from build123d import *

# Parameters (mm, degrees)
SKETCH2_W            = 53
SKETCH2_H            = 9
BOSS_EXTRUDE1_DEPTH  = 3
SKETCH11_W           = 2
SKETCH11_H           = 9
CUT_EXTRUDE3_DEPTH   = 5
SKETCH12_W           = 3
SKETCH12_H           = 9
BOSS_EXTRUDE7_DEPTH  = 1
SKETCH13_W           = 1
SKETCH13_H           = 1
BOSS_EXTRUDE8_DEPTH  = 4
SKETCH14_W           = 1
SKETCH14_H           = 1
BOSS_EXTRUDE9_DEPTH  = 5
SKETCH15_W           = 45.862173985
SKETCH15_H           = 3
BOSS_EXTRUDE10_DEPTH = 1.5
SKETCH25_W           = 3
SKETCH25_H           = 9
BOSS_EXTRUDE13_DEPTH = 1
SKETCH24_R           = 1.16794594
CUT_EXTRUDE7_DEPTH   = 9
SKETCH26_W           = 0.9784551
SKETCH26_H           = 1.939455742
CUT_EXTRUDE8_DEPTH   = 9
SKETCH27_W           = 45.862173985
SKETCH27_H           = 3
BOSS_EXTRUDE14_DEPTH = 2
SKETCH28_W           = 41.224865511
SKETCH28_H           = 1
CUT_EXTRUDE9_DEPTH   = 1.5
SKETCH29_W           = 3
SKETCH29_H           = 12.5
BOSS_EXTRUDE15_DEPTH = 1
BOSS_EXTRUDE16_DEPTH = 1
SKETCH31_W           = 2.328454802
SKETCH31_H           = 1
CUT_EXTRUDE10_DEPTH  = 1.5
BOSS_EXTRUDE17_DEPTH = 2
BOSS_EXTRUDE18_REACH = 53.942
SKETCH34_W           = 46.86
SKETCH34_H           = 1.5
SKETCH35_W           = 43.553320313
SKETCH35_H           = 1.25
CUT_EXTRUDE11_DEPTH  = 1
CUT_EXTRUDE12_REACH  = 54.259
SKETCH36_W           = 46.86
SKETCH36_H           = 3.75
SKETCH37_W           = 2
SKETCH37_H           = 2.25
CUT_EXTRUDE13_DEPTH  = 10
BOSS_EXTRUDE19_DEPTH = 2.5
SKETCH42_W           = 43.553320313
SKETCH42_H           = 1
BOSS_EXTRUDE20_DEPTH = 1
SKETCH44_W           = 46.862173985
SKETCH44_H           = 1
BOSS_EXTRUDE21_DEPTH = 5
SKETCH46_W           = 43.553320313
SKETCH46_H           = 1
BOSS_EXTRUDE22_DEPTH = 1


with BuildPart() as part:
    # Sketch2 → Boss-Extrude1 (new body)
    with BuildSketch(Plane.XY):
        with Locations((26.5, 4.5)):
            Rectangle(SKETCH2_W, SKETCH2_H)
    extrude(amount=BOSS_EXTRUDE1_DEPTH)

    # Sketch11 → Cut-Extrude3 (cut)
    with BuildSketch(Plane.XY.offset(3)):
        with Locations((52, 4.5)):
            Rectangle(SKETCH11_W, SKETCH11_H)
    extrude(amount=-CUT_EXTRUDE3_DEPTH, mode=Mode.SUBTRACT)

    # Sketch12 → Boss-Extrude7 (add)
    with BuildSketch(Plane.XY.offset(3)):
        with Locations((48, 4.5)):
            Rectangle(SKETCH12_W, SKETCH12_H)
    extrude(amount=BOSS_EXTRUDE7_DEPTH)

    # Sketch13 → Boss-Extrude8 (add)
    with BuildSketch(Plane.XY.offset(3)):
        with Locations((7, 7.5)):
            Rectangle(SKETCH13_W, SKETCH13_H)
        with Locations((7, 1.5)):
            Rectangle(SKETCH13_W, SKETCH13_H)
    extrude(amount=BOSS_EXTRUDE8_DEPTH)

    # Sketch14 → Boss-Extrude9 (add)
    with BuildSketch(Plane.XZ.offset(-7)):
        with Locations((7, 6.5)):
            Rectangle(SKETCH14_W, SKETCH14_H)
    extrude(amount=BOSS_EXTRUDE9_DEPTH)

    # Sketch15 → Boss-Extrude10 (add)
    with BuildSketch(Plane.XZ):
        with Locations((22.931086993, 1.5)):
            Rectangle(SKETCH15_W, SKETCH15_H)
    extrude(amount=BOSS_EXTRUDE10_DEPTH)

    # Sketch25 → Boss-Extrude13 (add)
    with BuildSketch(Plane(origin=(0, 0, 0), x_dir=(-1, 0, 0), z_dir=(0, 0, -1))):
        with Locations((-48, 4.5)):
            Rectangle(SKETCH25_W, SKETCH25_H)
    extrude(amount=BOSS_EXTRUDE13_DEPTH)

    # Sketch24 → Cut-Extrude7 (cut)
    with BuildSketch(Plane(origin=(0, 9, 0), x_dir=(1, 0, 0), z_dir=(0, 1, 0))):
        with Locations(Location((48, -2, 0), (0, 0, 270))):
            Circle(SKETCH24_R)
    extrude(amount=-CUT_EXTRUDE7_DEPTH, mode=Mode.SUBTRACT)

    # Sketch26 → Cut-Extrude8 (cut)
    with BuildSketch(Plane(origin=(0, 9, 0), x_dir=(1, 0, 0), z_dir=(0, 1, 0))):
        with Locations((48, 0.030272129)):
            Rectangle(SKETCH26_W, SKETCH26_H)
    extrude(amount=-CUT_EXTRUDE8_DEPTH, mode=Mode.SUBTRACT)

    # Sketch27 → Boss-Extrude14 (add)
    with BuildSketch(Plane.XZ.offset(1.5)):
        with Locations((22.931086993, 1.5)):
            Rectangle(SKETCH27_W, SKETCH27_H)
    extrude(amount=BOSS_EXTRUDE14_DEPTH)

    # Sketch28 → Cut-Extrude9 (cut)
    with BuildSketch(Plane.XZ.offset(3.5)):
        with Locations((22.921286428, 0.5)):
            Rectangle(SKETCH28_W, SKETCH28_H)
    extrude(amount=-CUT_EXTRUDE9_DEPTH, mode=Mode.SUBTRACT)

    # Sketch29 → Boss-Extrude15 (add)
    with BuildSketch(Plane.ZY):
        with Locations((1.5, 2.75)):
            Rectangle(SKETCH29_W, SKETCH29_H)
    extrude(amount=BOSS_EXTRUDE15_DEPTH)

    # Sketch30 → Boss-Extrude16 (add)
    with BuildSketch(Plane.ZY.offset(-6.5)):
        Polygon((3, 8), (3, 7), (6, 7), (6, 2), (3, 2), (3, 1), (7, 1), (7, 8), align=None)
    extrude(amount=BOSS_EXTRUDE16_DEPTH)

    # Sketch31 → Cut-Extrude10 (cut)
    with BuildSketch(Plane.XZ.offset(3.5)):
        with Locations((44.697946584, 0.5)):
            Rectangle(SKETCH31_W, SKETCH31_H)
    extrude(amount=-CUT_EXTRUDE10_DEPTH, mode=Mode.SUBTRACT)

    # Sketch32 → Boss-Extrude17 (add)
    with BuildSketch(Plane.XZ.offset(3.5)):
        Polygon((-1, 3), (-1, 0), (2.308853672, 0), (2.308853672, 1), (45.862173985, 1), (45.862173985, 3), align=None)
    extrude(amount=BOSS_EXTRUDE17_DEPTH)

    # Boss-Extrude18: up to this face of the body (flat: up to its plane)
    boss_extrude18_end = Plane(part.part.faces().sort_by_distance((22.213634354, 3.353188918, 0))[0])
    # Sketch34 → Boss-Extrude18 (add, up to the picked face)
    with BuildSketch(Plane.XY.offset(3), mode=Mode.PRIVATE) as boss_extrude18_sk1:
        with Locations((22.43, -6.25)):
            Rectangle(SKETCH34_W, SKETCH34_H)
    boss_extrude18_tool1 = split(extrude(boss_extrude18_sk1.sketch, amount=-BOSS_EXTRUDE18_REACH, mode=Mode.PRIVATE), bisect_by=boss_extrude18_end, keep=Keep.BOTH, mode=Mode.PRIVATE)
    add(boss_extrude18_tool1.solids().sort_by(Axis((22.43, -6.25, 3), (0, 0, -1)))[0])

    # Sketch35 → Cut-Extrude11 (cut)
    with BuildSketch(Plane(origin=(0, 0, 0), x_dir=(-1, 0, 0), z_dir=(0, 0, -1))):
        with Locations((-24.085513829, -1.375)):
            Rectangle(SKETCH35_W, SKETCH35_H)
    extrude(amount=-CUT_EXTRUDE11_DEPTH, mode=Mode.SUBTRACT)

    # Cut-Extrude12: up to this face of the body (flat: up to its plane)
    cut_extrude12_end = Plane(part.part.faces().sort_by_distance((50.25, 4.5, 3))[0])
    # Sketch36 → Cut-Extrude12 (cut, up to the picked face)
    with BuildSketch(Plane(origin=(0, 0, 0), x_dir=(-1, 0, 0), z_dir=(0, 0, -1)), mode=Mode.PRIVATE) as cut_extrude12_sk1:
        with Locations((-22.43, -5.125)):
            Rectangle(SKETCH36_W, SKETCH36_H)
    cut_extrude12_tool1 = split(extrude(cut_extrude12_sk1.sketch, amount=-CUT_EXTRUDE12_REACH, mode=Mode.PRIVATE), bisect_by=cut_extrude12_end, keep=Keep.BOTH, mode=Mode.PRIVATE)
    add(cut_extrude12_tool1.solids().sort_by(Axis((22.43, -5.125, 0), (0, 0, 1)))[0], mode=Mode.SUBTRACT)

    # Sketch37 → Cut-Extrude13 (cut)
    with BuildSketch(Plane.ZY.offset(-45.86)):
        with Locations((2, -4.375)):
            Rectangle(SKETCH37_W, SKETCH37_H)
    extrude(amount=-CUT_EXTRUDE13_DEPTH, mode=Mode.SUBTRACT)

    # Sketch41 → Boss-Extrude19 (add)
    with BuildSketch(Plane.XZ.offset(3.25)):
        Polygon((-1, 0), (-1, 3), (45.862173985, 3), (45.862173985, 1), (2.308853672, 1), (2.308853672, 0), align=None)
    extrude(amount=BOSS_EXTRUDE19_DEPTH)

    # Sketch42 → Boss-Extrude20 (add)
    with BuildSketch(Plane(origin=(0, 0, 1), x_dir=(-1, 0, 0), z_dir=(0, 0, -1))):
        with Locations((-24.085513829, -5.25)):
            Rectangle(SKETCH42_W, SKETCH42_H)
    extrude(amount=BOSS_EXTRUDE20_DEPTH)

    # Sketch44 → Boss-Extrude21 (add)
    with BuildSketch(Plane(origin=(0, 0, 0), x_dir=(-1, 0, 0), z_dir=(0, 0, -1))):
        with Locations((-22.431086993, -5.25)):
            Rectangle(SKETCH44_W, SKETCH44_H)
    extrude(amount=BOSS_EXTRUDE21_DEPTH)

    # Sketch46 → Boss-Extrude22 (add)
    with BuildSketch(Plane.XZ.offset(0.75)):
        with Locations((24.085513829, 0.5)):
            Rectangle(SKETCH46_W, SKETCH46_H)
    extrude(amount=BOSS_EXTRUDE22_DEPTH)


solid = part.part
Input: part model. Units: mm. Frame: model coordinates. A direction names the side the tool comes from. Coordinates: 2 decimals unless noted, no trailing zeros. Loops run counter-clockwise (first coordinate to the right, second up) from the corner with the lowest first, then second, coordinate; pieces in that order, holes last. Notation, with made-up numbers: (89, 52.5) -> (144, 52.5) arc R6 ccw to (144, 63.5) -> close; hole circle Ø3 at (-28, -21.5). An arc over 180 degrees is marked (long way). Write each question's results on one line, items separated by ' | '. Start each with the question number.
Q1. Pin query (flat end, axial travel): pin 1 (1.5 mm diameter, centred on x = 48, y = 6.5, fed in from +Z); pin 2 (1 mm diameter, centred on x = 6, z = 4.5, fed in from +Y); pin 3 (0.5 mm diameter, centred on y = 5, z = 3.5, fed in from -X). Return the tip coordinate at first contact, or that it passes through.
Q2. Pull-direction query (X, two-part tool) for faces 4 (the flat face through (7, 8, 5)), 5 (the cylindrical face through (47.956, 4.563, 3.167)), 6 (the flat face through (48.489, 5, 0)), 7 (the flat face through (-1, 0, 1)); classes: released by +X, released by -X, zero draft, split by the parting line, or undercut.
Q3. Section C-C, the plane x = 31.5. Return the cut outline in (y, z).
Q4. Section A-A, the plane y = 5. Return the cut outline in (x, z), plus the area to 3 significant figures.
Q5. Reachability of faces 1 (the flat face through (7, 7, 4)), 2 (the flat face through (48, 5, 4)), 3 (the flat face through (49, 0, 1)) from +Z, -Z, +X, -X, +Y, -Y: full face, straight path, thin tool, end or side. Return the list, or none.
Q6. Section B-B, the plane z = 2. Return the cut outline in (x, y), plus the area to 3 significant figures.
Q7. Section D-D, the plane y = -0.5. Return the cut outline in (x, z).
Q8. Ray query, line 1 (X direction, y = 2.5, z = 2); line 2 (Z direction, x = 48, y = 5.5); line 3 (Z direction, x = 32, y = 7). Return the intervals inside material, ascending. Write a range as from..to.
Found:
1) pin 1: z = 4 | pin 2: y = 8 | pin 3: x = 46.5
2) face 4: zero draft | face 5: undercut | face 6: undercut | face 7: released by -X
3) outline: (-5.75, -5) -> (-4.75, -5) -> (-4.75, 1) -> (-1.75, 1) -> (-1.75, 0) -> (9, 0) -> (9, 3) -> (-5.75, 3) -> close
4) outline: (-1, 0) -> (46.5, 0) -> (46.5, -1) -> (47.51, -1) -> (47.51, 0.94) arc R1.17 cw (long way) to (48.49, 0.94) -> (48.49, -1) -> (49.5, -1) -> (49.5, 0) -> (51, 0) -> (51, 3) -> (49.5, 3) -> (49.5, 4) -> (46.5, 4) -> (46.5, 3) -> (-1, 3) -> close; (5.5, 6) -> (7.5, 6) -> (7.5, 7) -> (5.5, 7) -> close | area: 158 mm2
5) face 1: -X | face 2: +Z, +X, +Y, -Y | face 3: +Z, -Z, +X, -Y
6) outline: (-1, -5.75) -> (45.86, -5.75) -> (45.86, 0) -> (46.83, 0) -> (46.83, 9) -> (-1, 9) -> close; (49.17, 0) -> (51, 0) -> (51, 9) -> (49.17, 9) -> close | area: 716 mm2
7) outline: (-1, 0) -> (45.86, 0) -> (45.86, 3) -> (-1, 3) -> close
8) line 1: -1..46.83, 49.17..51 | line 2: 3.17..4 | line 3: 0..3
